Part print with two shaded views. Sizes in mm from the minimum x, y, z corner. Coordinates: 2 decimals unless noted, no trailing zeros. Order: outer loops, then holes, each group sorted by start corner. A loop starts at its lowest first (then second) coordinate and runs counter-clockwise, first axis right, second up. Notation, with made-up numbers: (82, 43.5) - (95, 43.5) arc R20 ccw to (95, 53.5) - close; hole circle Ø4 at (42.25, 73.5). An arc over 180 degrees is marked (long way). One line per item, written item: value.
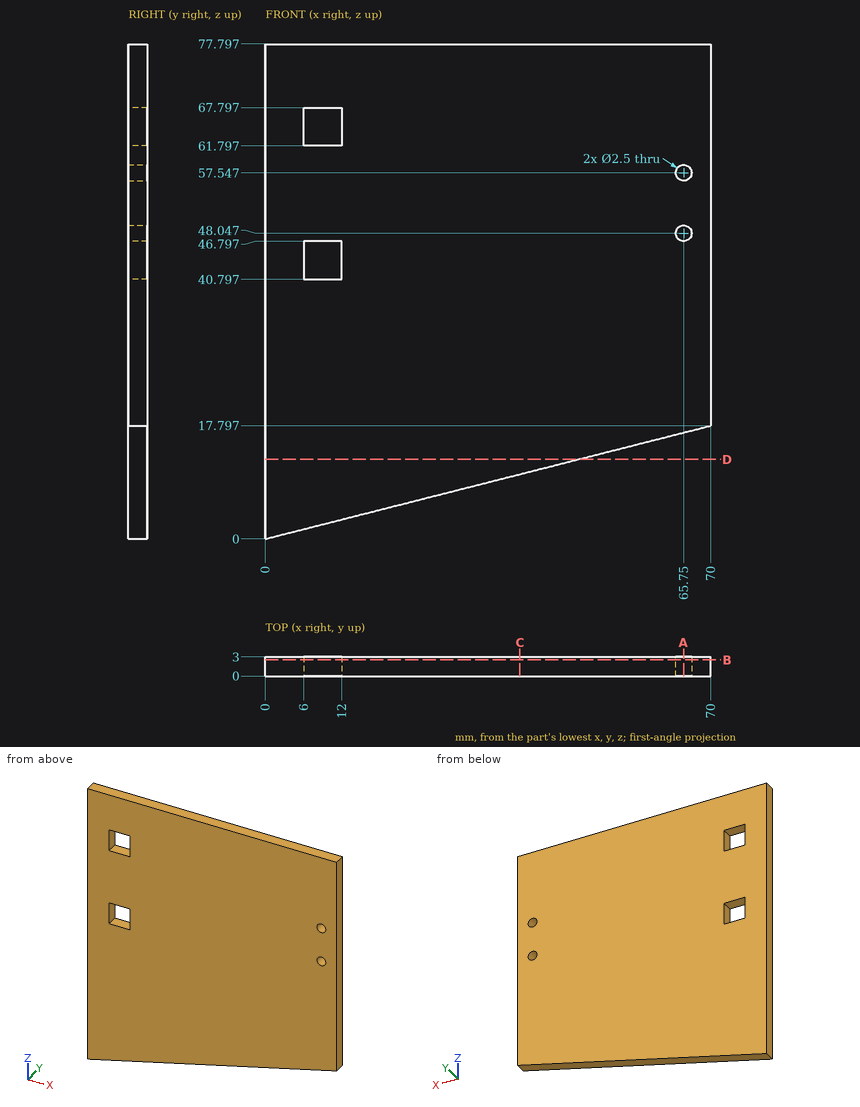
1. Band-saw the part on B-B, the plane y = 2.55. Give the cut face in (x, z).
Values found:
outline: (0, 0) - (70, 17.8) - (70, 77.8) - (0, 77.8) - close; hole (6, 40.8) - (12, 40.8) - (12, 46.8) - (6, 46.8) - close; hole (6, 61.8) - (12, 61.8) - (12, 67.8) - (6, 67.8) - close; hole circle Ø2.5 at (65.75, 48.05); hole circle Ø2.5 at (65.75, 57.55)
2. Flat gauge pins, fed straight in: P1, Ø0.9, axis at y = 2, z = 42.5, coming from the -X side; P2, Ø0.9, axis at x = 10.5, y = 1.5, coming from the -Z side (1 decimal). Where does each tip first touch, or does it go through?
Values found:
P1: stops at x = 0
P2: stops at z = 2.6
3. Band-saw the part on A-A, the plane x = 65.75. Give the cut face in (y, z), and give its area (3 significant figures).
Values found:
outline: (0, 16.72) - (3, 16.72) - (3, 46.8) - (0, 46.8) - close; (0, 49.3) - (3, 49.3) - (3, 56.3) - (0, 56.3) - close; (0, 58.8) - (3, 58.8) - (3, 77.8) - (0, 77.8) - close
area: 168 mm2
4. Band-saw the part on C-C, the plane x = 40. Give the cut face in (y, z).
Values found:
outline: (0, 10.17) - (3, 10.17) - (3, 77.8) - (0, 77.8) - close
5. Probe line 1 along Z through (x, y) = (8, 0.5) (1 decimal); line 2 along Z through (x, y) = (66.5, 0.85) (1 decimal); line 3 along X through (y, z) = (2.4, 63.5). List the from-to ranges inside material, lowest first.
Values found:
line 1: z = 2 to 40.8, 46.8 to 61.8, 67.8 to 77.8
line 2: z = 16.9 to 47, 49 to 56.5, 58.5 to 77.8
line 3: x = 0 to 6, 12 to 70
6. Band-saw the part on D-D, the plane z = 12.5. Give the cut face in (x, y).
Values found:
outline: (0, 0) - (49.17, 0) - (49.17, 3) - (0, 3) - close
